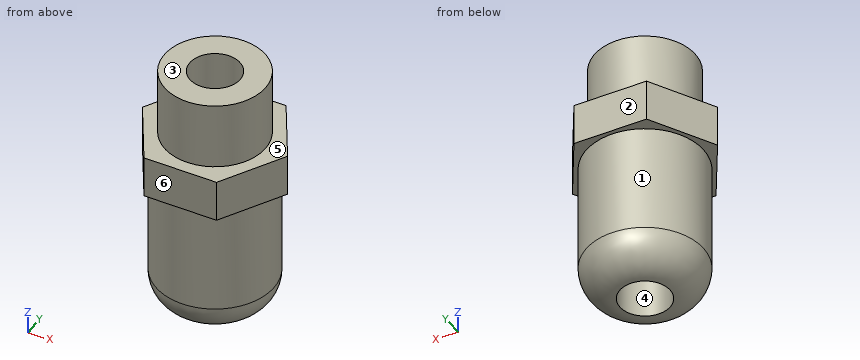
from build123d import *

# Parameters (mm, degrees)
SKICA1_R                 = 6
P_IDAT_VYSUNUT_M1_DEPTH  = 8
P_IDAT_VYSUNUT_M2_DEPTH  = 5
SKICA3_R                 = 7
P_IDAT_VYSUNUT_M3_DEPTH  = 17
ZAOBLIT1_R               = 4
SKICA4_R                 = 3
ODEBRAT_VYSUNUT_M1_DEPTH = 33.113081447


with BuildPart() as part:
    # Skica1 → Přidat vysunutím1 (new body)
    with BuildSketch(Plane.XY):
        Circle(SKICA1_R)
    extrude(amount=P_IDAT_VYSUNUT_M1_DEPTH)

    # Skica2 → Přidat vysunutím2 (add)
    with BuildSketch(Plane(origin=(0, 0, 0), x_dir=(-1, 0, 0), z_dir=(0, 0, -1))):
        Polygon((4.330127019, -7.5), (8.660254038, 0), (4.330127019, 7.5), (-4.330127019, 7.5), (-8.660254038, 0), (-4.330127019, -7.5), align=None)
    extrude(amount=P_IDAT_VYSUNUT_M2_DEPTH)

    # Skica3 → Přidat vysunutím3 (add)
    with BuildSketch(Plane(origin=(0, 0, -5), x_dir=(-1, 0, 0), z_dir=(0, 0, -1))):
        Circle(SKICA3_R)
    extrude(amount=P_IDAT_VYSUNUT_M3_DEPTH)

    # Zaoblit1
    zaoblit1_edges = [part.edges().sort_by_distance(p)[0] for p in [
        (7, 0, -22),
    ]]
    fillet(zaoblit1_edges, radius=ZAOBLIT1_R)

    # Skica4 → Odebrat vysunutím1 (cut, through all)
    with BuildSketch(Plane.XY.offset(8)):
        Circle(SKICA4_R)
    extrude(amount=-ODEBRAT_VYSUNUT_M1_DEPTH, mode=Mode.SUBTRACT)


solid = part.part
The listing builds one solid part. Answer for the finished solid, in the listing's coordinates (mm). Face numbers are marked on the shaded views. A direction names the side the tool comes from. Round coordinates to 2 decimals unless told otherwise and drop trailing zeros. Order: outer loops, then holes, each group sorted by start corner. A loop starts at its lowest first (then second) coordinate and runs counter-clockwise, first axis right, second up. Notation, with made-up numbers: (34, -1) - (55, -1) arc R25 cw to (55, 18) - close; hole circle Ø2 at (48, 80.25). An arc over 180 degrees is marked (long way). Write item = value, one per line. Start each with the question number.
1) Given pin 1 (2 mm diameter, centred on x = -1.5, z = -16.5, fed in from -Y); pin 2 (2 mm diameter, centred on y = -1.5, z = -15.5, fed in from +X); pin 3 (5 mm diameter, centred on x = -3, z = -17, fed in from +Y), each flat-ended and moving along its own axis, determine where each tip first touches the part or whether it passes through.
2) Section C-C, the plane x = 7.5 is taken. Write down the section's boundary in (y, z).
3) Straight lines are drawn through the part: L1, parallel to Y at x = 0, z = -8.75; L2, parallel to X at y = -0.5, z = -10.5; L3, parallel to Z at x = -7, y = 1.25. For each, find the intervals that lie inside material, in ascending order.
4) For a pull along Y with two mould halves and no side action, classify the marked faces 1, 2, 3 and 4 as released by +Y, released by -Y, zero draft, split by the parting line, or undercut.
5) Section A-A, the plane z = 2.5 is taken. Write down the section's boundary in (x, y).
6) Section B-B, the plane z = -7.5 is taken. Write down the section's boundary in (x, y), plus the area to 3 significant figures.
7) For the marked faces 5 and 6, determine the directions among +Z, -Z, +X, -X, +Y, -Y from which every point of the face is accessible in a straight line to the end or side of a thin tool.
Results list:
q1.pin_1 = -6.98
q1.pin_2 = 6.98
q1.pin_3 = 6.98
q2.outline = (-2.01, -5) - (2.01, -5) - (2.01, 0) - (-2.01, 0) - close
q3.L1 = -7 to -3, 3 to 7
q3.L2 = -6.98 to -2.96, 2.96 to 6.98
q3.L3 = -5 to 0
q4.face_1 = split by the parting line
q4.face_2 = released by +Y
q4.face_3 = zero draft
q4.face_4 = undercut
q5.outline = circle Ø12 at (0, 0); hole circle Ø6 at (0, 0)
q6.outline = circle Ø14 at (0, 0); hole circle Ø6 at (0, 0)
q6.area = 126 mm^2
q7.face_5 = +Z
q7.face_6 = +Z, -Z, +X, -X, -Y
